```python
from build123d import *

# Parameters (mm, degrees)
F1_DEPTH = 25
F2_R     = 12.49999


# Not quite as in the source:
# - a fillet or chamfer is up to 0.001 mm smaller than in the source, because OpenCascade refuses the exact size


with BuildPart() as f1:
    # F0 (on Front) → F1 (new body)
    with BuildSketch(Plane.XZ):
        with BuildLine():
            Line((-277.959928672, -3.7163552741), (-277.959928672, -123.7163552741))
            Line((-277.959928672, -123.7163552741), (-27.959928672, -123.7163552741))
            Line((-27.959928672, -123.7163552741), (-27.959928672, -3.7163552741))
            Line((-27.959928672, -3.7163552741), (-43.9558270226, -3.7163552741))
            ThreePointArc((-43.9558270226, -3.7163552741), (-152.9567080066, -67.529690512), (-261.9575889906, -3.7163552741))
            Line((-261.9575889906, -3.7163552741), (-277.959928672, -3.7163552741))
        make_face()
    extrude(amount=F1_DEPTH)

    # F2 (radius 12.5 in the source; OpenCascade refuses exactly that, so slightly less here)
    f2_edges = [f1.edges().sort_by_distance(p)[0] for p in [
        (-261.957589, -12.5, -3.716355),
        (-43.955827, -12.5, -3.716355),
        (-152.956708, -25, -67.529691),
        (-152.956708, 0, -67.529691),
    ]]
    fillet(f2_edges, radius=F2_R)


solid = f1.part
```
Can you work these out from the model? Positions are in its coordinate system, mm. A direction names the side the tool comes from. Give positions to 0.01 mm unless a question says otherwise; leave off trailing zeros. Loops run counter-clockwise (first coordinate to the right, second up) from the corner with the lowest first, then second, coordinate; pieces in that order, holes last. Notation, with made-up numbers: M 26.5,40.25 L 33.5,40.25 A19 cw 33.5,58.25 Z; hole C 50.5,-10.75 d9. An arc over 180 degrees is marked long. Use one line per item in the form item = value. Start each with the question number.
(1) I want a section at A-A, the plane y = -18.5. Write out the boundary of the cut face in (x, z).
(2) Please list where these lines run through material, in increasing order: line 1 (Y direction, x = -152.5, z = -79.5); line 2 (X direction, y = -1.75, z = -38.5); line 3 (Y direction, x = -68, z = -37).
(3) I'm going to push a flat-ended pin straight in: P1, Ø3, axis at x = -111, y = -12.5, coming from the +Z side. Where does the tip first touch, or does it pass through?
(4) On a 3-axis mill with a long thin cutter (end or side, diameter ignored), from which of +Z, -Z, +X, -X, +Y, -Y can I reach the whole of each face in a straight line? I mean faces 1 (the cylindrical face through (-41.55, -12.651, -4.626)), 2 (the flat face through (-32, -12, -3.716)). Say none if no direction works.
(5) Thinking about a two-plate mould opening in X: for faces 3 (the flat face through (-155, 0, -90)), 4 (the flat face through (-27.96, -12, -65)), 5 (the cylindrical face through (-264.201, -12.651, -4.693)), 6 (the flat face through (-277.96, -12, -63)), which applies, released by +X, released by -X, zero draft, split by the parting line, or undercut?
(6) I want a section at B-B, the plane y = -5.5. Write out the boundary of the cut face in (x, z), and give its area (3 significant figures).
Worked out:
q1.outline = M -277.96,-123.72 L -27.96,-123.72 L -27.96,-3.72 L -36.87,-3.72 A12.5 ccw -43.15,-5.41 A126.53 cw -262.76,-5.41 A12.5 ccw -269.05,-3.72 L -277.96,-3.72 Z
q2.line_1 = -24.99 to -0.01
q2.line_2 = -277.96 to -242.3, -63.61 to -27.96
q2.line_3 = -19.36 to -5.64
q3.P1 = -59.73
q4.face_1 = +Z, +Y, -Y
q4.face_2 = +Z, +X, -X, +Y, -Y
q5.face_3 = zero draft
q5.face_4 = released by +X
q5.face_5 = undercut
q5.face_6 = released by -X
q6.outline = M -277.96,-123.72 L -27.96,-123.72 L -27.96,-3.72 L -36.87,-3.72 A12.5 ccw -42.16,-4.89 A127.14 cw -263.76,-4.89 A12.5 ccw -269.05,-3.72 L -277.96,-3.72 Z
q6.area = 19,500 mm²
